Work out the finished part from the listing and answer in its coordinate system (mm). Round coordinates to 2 decimals unless told otherwise and drop trailing zeros. Order: outer loops, then holes, each group sorted by start corner. A loop starts at its lowest first (then second) coordinate and runs counter-clockwise, first axis right, second up.
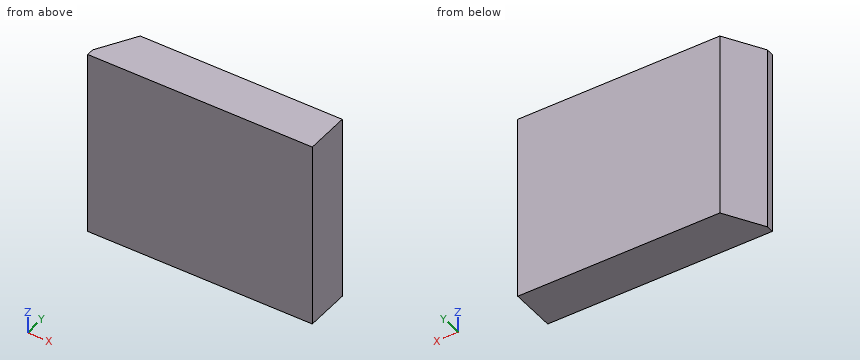
from build123d import *

# Parameters (mm, degrees)
SKETCH1_W           = 60
SKETCH1_H           = 12
BOSS_EXTRUDE1_DEPTH = 50
CUT_EXTRUDE1_DEPTH  = 80.018985061


with BuildPart() as part:
    # Sketch1 → Boss-Extrude1 (new body)
    with BuildSketch(Plane.XY):
        with Locations((30, 6)):
            Rectangle(SKETCH1_W, SKETCH1_H)
    extrude(amount=BOSS_EXTRUDE1_DEPTH)

    # Sketch2 → Cut-Extrude1 (cut, through all)
    with BuildSketch(Plane.XY.offset(50)):
        Polygon((0, 2), (6, 12), (0, 12), align=None)
    extrude(amount=-CUT_EXTRUDE1_DEPTH, mode=Mode.SUBTRACT)


solid = part.part
Item 1: Find section A-A (z = 21). Write down the section's boundary in (x, y), plus the area to 3 significant figures.
Item 2: Given pin 1 (2 mm diameter, centred on x = 46.5, y = 6, fed in from -Z); pin 2 (4 mm diameter, centred on y = 9.5, z = 21.5, fed in from -X), each flat-ended and moving along its own axis, determine where each tip first touches the part or whether it passes through.
Item 3: Find section C-C (y = 10.5). Write down the section's boundary in (x, z).
Item 4: Find section B-B (y = 7). Write down the section's boundary in (x, z).
Item 5: Find the intervals of material crossed by line 1 along X through (y, z) = (8.75, 28); line 2 along X through (y, z) = (2.5, 43.5), in increasing order.
Model answer:
1. outline: (0, 0) - (60, 0) - (60, 12) - (6, 12) - (0, 2) - close
1. area: 690 mm2
2. pin 1: stops at z = 0
2. pin 2: stops at x = 3.3
3. outline: (5.1, 0) - (60, 0) - (60, 50) - (5.1, 50) - close
4. outline: (3, 0) - (60, 0) - (60, 50) - (3, 50) - close
5. line 1: x = 4.05 to 60
5. line 2: x = 0.3 to 60
